Design review of the part built by this model. Coordinates are the model's own, in mm. A direction names the side the tool comes from. Coordinates: 2 decimals unless noted, no trailing zeros. Write each loop counter-clockwise with the first axis right and the second up, starting at its lowest first coordinate (ties: lowest second). Pieces come first, ordered by that corner, then holes. Notation, with made-up numbers: (-15, 62) - (13, 62) arc R30 cw to (13, 84) - close; hole circle Ø6 at (38.5, 49). An arc over 180 degrees is marked (long way). Use a Markdown table: item, result.
from build123d import *

# Parameters (mm, degrees)
FILETE2_R             = 0.5
FILETE3_R             = 0.5
FILETE4_R             = 0.5
FILETE5_R             = 0.5
ESBO_O5_R             = 1
CORTE_EXTRUS_O1_DEPTH = 3
CHANFRO1_SIZE         = 1


with BuildPart() as part:
    # Esboço1 → Revolução1 (revolve)
    with BuildSketch(Plane.XY):
        Polygon((0, 5), (0, 10.27), (4, 10.27), (4, 7.77), (6.62, 7.77), (6.62, 10.27), (9.62, 10.27), (9.62, 5.8), (15.87, 5.8), (15.87, 2.3), (24.87, 2.3), (25.87, 1.3), (25.87, 0), (9.386751346, 0), (6.5, 5), align=None)
    revolve(axis=Axis((25.87, 0, 0), (-1, 0, 0)))

    # Filete2
    filete2_edges = [part.edges().sort_by_distance(p)[0] for p in [
        (0, -5, 0),
    ]]
    fillet(filete2_edges, radius=FILETE2_R)

    # Filete3
    filete3_edges = [part.edges().sort_by_distance(p)[0] for p in [
        (0, -10.27, 0),
    ]]
    fillet(filete3_edges, radius=FILETE3_R)

    # Filete4
    filete4_edges = [part.edges().sort_by_distance(p)[0] for p in [
        (9.62, -10.27, 0),
    ]]
    fillet(filete4_edges, radius=FILETE4_R)

    # Filete5
    filete5_edges = [part.edges().sort_by_distance(p)[0] for p in [
        (15.87, -5.8, 0),
    ]]
    fillet(filete5_edges, radius=FILETE5_R)

    # Esboço5 → Corte-extrusão1 (cut)
    with BuildSketch(Plane(origin=(0, 0, -10.27), x_dir=(-1, 0, 0), z_dir=(0, 0, -1))):
        with Locations((-2, 0)):
            Circle(ESBO_O5_R)
    extrude(amount=-CORTE_EXTRUS_O1_DEPTH, mode=Mode.SUBTRACT)

    # Chanfro1
    chanfro1_edges = [part.edges().sort_by_distance(p)[0] for p in [
        (3, 0, -7.27),
    ]]
    chamfer(chanfro1_edges, length=CHANFRO1_SIZE)


solid = part.part
(1) Machinability: for faces 1 (the cylindrical face through (3.46, -1.08, 4.88)), 2 (the flat face through (6.62, 2, -8)), 3 (the cylindrical face through (2.8, -0.6, -9.3)), 4 (the flat face through (9.62, 4.21, 4.21)), which of the approach directions +Z, -Z, +X, -X, +Y, -Y give a long, thin tool a straight path to every point of the face, cutting with its end or side? Answer none if there is none.
Determined:
| item | result |
|---|---|
| face 1 | -X |
| face 2 | none |
| face 3 | -Z |
| face 4 | +X |
(2) For L1, parallel to X at y = 0, z = -8.95; L2, parallel to X at y = 6.5, z = -6; L3, parallel to X at y = -3.5, z = 5, list the stretches that pass through material, from the lowest coordinate up. Write a range as from..to.
Determined:
| item | result |
|---|---|
| L1 | 0..1, 3..4, 6.62..9.62 |
| L2 | 0..4, 6.62..9.62 |
| L3 | 0..9.62 |
(3) Take a section at B-B on x = 13.5. Write out the cut boundary in (y, z), and give its area (3 significant figures).
Determined:
| item | result |
|---|---|
| outline | circle Ø11.6 at (0, 0) |
| area | 106 mm2 |
(4) Draft analysis for pull direction X (two halves, no side actions). For faces 5 (the flat face through (25.87, 0, 0)), 6 (the cylindrical face through (12.535, -5.794, -0.255)), 7 (the cylindrical face through (5.328, 7.411, -2.334)), 8 (the flat face through (0, -4, 4)), state which applies: +X half, -X half, draft (parallel to the pull), parting line (faces both ways), or undercut.
Determined:
| item | result |
|---|---|
| face 5 | +X half |
| face 6 | draft |
| face 7 | undercut |
| face 8 | -X half |
(5) For pin 1 (12 mm diameter, centred on x = 17.5, z = 2.5, fed in from +Y); pin 2 (1.5 mm diameter, centred on x = 8, y = -6.5, fed in from +Z); pin 3 (1 mm diameter, centred on y = 7.5, z = -6, fed in from +X), all flat-tipped, find the tip position at first contact; note any pin that passes through.
Determined:
| item | result |
|---|---|
| pin 1 | y = 5.8 |
| pin 2 | z = 8.51 |
| pin 3 | x = 9.62 |
(6) Take a section at A-A on x = 21.25. Write out the cut boundary in (y, z).
Determined:
| item | result |
|---|---|
| outline | circle Ø4.6 at (0, 0) |
